```python
from build123d import *

# Parameters (mm, degrees)
BOSS_EXTRUDE1_DEPTH = 2
SKETCH1_3_W         = 42
SKETCH1_3_H         = 2
SKETCH1_3_W_2       = 9
BOSS_EXTRUDE2_DEPTH = 23
FILLET1_R           = 2
SKETCH2_R           = 1.5
CUT_EXTRUDE1_DEPTH  = 25
SKETCH3_R           = 2
SKETCH3_R_2         = 4
SKETCH3_R_3         = 1.5
CUT_EXTRUDE2_DEPTH  = 25
SKETCH4_R           = 2
CUT_EXTRUDE3_DEPTH  = 25


with BuildPart() as part:
    # Sketch1 → Boss-Extrude1 (new body)
    with BuildSketch(Plane.XY):
        with BuildLine():
            Line((-21, -18.5), (21, -18.5))
            Line((21, -18.5), (21, -10.5))
            Line((21, -10.5), (27, -10.5))
            ThreePointArc((27, -10.5), (28.414213562, -9.914213562), (29, -8.5))
            Line((29, -8.5), (29, 14.5))
            Line((29, 14.5), (20, 14.5))
            Line((20, 14.5), (20, 8.5))
            Line((20, 8.5), (18, 8.5))
            Line((18, 8.5), (18, 16.5))
            ThreePointArc((18, 16.5), (17.414213562, 17.914213562), (16, 18.5))
            Line((16, 18.5), (-16, 18.5))
            ThreePointArc((-16, 18.5), (-17.414213562, 17.914213562), (-18, 16.5))
            Line((-18, 16.5), (-18, 8.5))
            Line((-18, 8.5), (-20, 8.5))
            Line((-20, 8.5), (-20, 14.5))
            Line((-20, 14.5), (-29, 14.5))
            Line((-29, 14.5), (-29, -8.5))
            ThreePointArc((-29, -8.5), (-28.414213562, -9.914213562), (-27, -10.5))
            Line((-27, -10.5), (-21, -10.5))
            Line((-21, -10.5), (-21, -18.5))
        make_face()
    extrude(amount=-BOSS_EXTRUDE1_DEPTH)

    # Sketch1<3> → Boss-Extrude2 (add)
    with BuildSketch(Plane.XY):
        with Locations((0, -17.5)):
            Rectangle(SKETCH1_3_W, SKETCH1_3_H)
        with Locations((-24.5, 13.5)):
            Rectangle(SKETCH1_3_W_2, SKETCH1_3_H)
        with Locations((24.5, 13.5)):
            Rectangle(SKETCH1_3_W_2, SKETCH1_3_H)
    extrude(amount=BOSS_EXTRUDE2_DEPTH)

    # Fillet1
    fillet1_edges = [part.edges().sort_by_distance(p)[0] for p in [
        (0, -18.5, -2),
        (24.5, 14.5, -2),
        (21, -17.5, 23),
        (-21, -17.5, 23),
        (-29, 13.5, 23),
        (-20, 13.5, 23),
        (20, 13.5, 23),
        (29, 13.5, 23),
        (-24.5, 14.5, -2),
    ]]
    fillet(fillet1_edges, radius=FILLET1_R)

    # Sketch2 → Cut-Extrude1 (cut)
    with BuildSketch(Plane(origin=(0, -16.5, 0), x_dir=(1, 0, 0), z_dir=(0, 1, 0))):
        with Locations((17.5, -11)):
            Circle(SKETCH2_R)
        with Locations((10.5, -11)):
            Circle(SKETCH2_R)
        with Locations((10.5, -18)):
            Circle(SKETCH2_R)
        with Locations((3.5, -11)):
            Circle(SKETCH2_R)
        with Locations((10.5, -4)):
            Circle(SKETCH2_R)
        with Locations((-17.5, -11)):
            Circle(SKETCH2_R)
        with Locations((-10.5, -18)):
            Circle(SKETCH2_R)
        with Locations((-10.5, -11)):
            Circle(SKETCH2_R)
        with Locations((-3.5, -11)):
            Circle(SKETCH2_R)
        with Locations((-10.5, -4)):
            Circle(SKETCH2_R)
    extrude(amount=-CUT_EXTRUDE1_DEPTH, mode=Mode.SUBTRACT)

    # Sketch3 → Cut-Extrude2 (cut)
    with BuildSketch(Plane.XY):
        with Locations((-24, -4.5)):
            Circle(SKETCH3_R)
        with Locations((-24, 5.5)):
            Circle(SKETCH3_R)
        with Locations((-10, 6.5)):
            Circle(SKETCH3_R_2)
        with Locations((-3, 6.5)):
            Circle(SKETCH3_R_3)
        with Locations((-10, -0.5)):
            Circle(SKETCH3_R_3)
        with Locations((-17, 6.5)):
            Circle(SKETCH3_R_3)
        with Locations((-10, 13.5)):
            Circle(SKETCH3_R_3)
        with Locations((10, -0.5)):
            Circle(SKETCH3_R_3)
        with Locations((3, 6.5)):
            Circle(SKETCH3_R_3)
        with Locations((10, 13.5)):
            Circle(SKETCH3_R_3)
        with Locations((10, 6.5)):
            Circle(SKETCH3_R_2)
        with Locations((17, 6.5)):
            Circle(SKETCH3_R_3)
        with Locations((24, -4.5)):
            Circle(SKETCH3_R)
        with Locations((24, 5.5)):
            Circle(SKETCH3_R)
        with Locations((0, -4.5)):
            Circle(SKETCH3_R_2)
        with Locations((0, -11.5)):
            Circle(SKETCH3_R_3)
        with Locations((-7, -4.5)):
            Circle(SKETCH3_R_3)
        with Locations((0, 2.5)):
            Circle(SKETCH3_R_3)
        with Locations((7, -4.5)):
            Circle(SKETCH3_R_3)
    extrude(amount=-CUT_EXTRUDE2_DEPTH, mode=Mode.SUBTRACT)

    # Sketch4 → Cut-Extrude3 (cut)
    with BuildSketch(Plane(origin=(0, 14.5, 0), x_dir=(1, 0, 0), z_dir=(0, 1, 0))):
        with Locations((-24, -7)):
            Circle(SKETCH4_R)
        with Locations((-24, -17)):
            Circle(SKETCH4_R)
        with Locations((24, -17)):
            Circle(SKETCH4_R)
        with Locations((24, -7)):
            Circle(SKETCH4_R)
    extrude(amount=-CUT_EXTRUDE3_DEPTH, mode=Mode.SUBTRACT)


solid = part.part
```
Verification items for the finished model (mm, model axes). A direction names the side the tool comes from. Give positions to 0.01 mm unless a question says otherwise; leave off trailing zeros. Order: outer loops, then holes, each group sorted by start corner. A loop starts at its lowest first (then second) coordinate and runs counter-clockwise, first axis right, second up. Notation, with made-up numbers: (19, -8.75) -> (32, -8.75) arc R19 ccw to (32, 10.25) -> close; hole circle Ø6 at (30, 9). An arc over 180 degrees is marked (long way). One line per item, written item: value.
(1) Gauge pin test, flat ends, axial feed: pin 1 (5 mm diameter, centred on x = -24, y = 5.5, fed in from +Z); pin 2 (3.5 mm diameter, centred on x = -10.5, z = 11, fed in from +Y); pin 3 (1 mm diameter, centred on x = 25, z = -0.5, fed in from -Y); pin 4 (2.5 mm diameter, centred on x = 10.5, z = 4, fed in from -Y). Record the tip position at first contact, or that the pin passes through.
Final values:
pin 1: z = 0
pin 2: y = -16.5
pin 3: y = -10.5
pin 4: through
(2) Tool access check on faces 1 (the face through (24.44, 13.93, -1.4)), 2 (the face through (20.57, 13.51, 22.4)), 3 (the face through (19, 8.5, -1)). Record the directions out of +Z, -Z, +X, -X, +Y, -Y that give a thin tool (end or side, any length) a straight path to the whole face; none if there is none.
Final values:
face 1: -Z, +X, +Y
face 2: +Z, +Y
face 3: +Z, -Z, +Y
(3) Sectioned sample at B-B on x = -24. Record the cut outline in (y, z), then the cut area to 3 significant figures.
Final values:
outline: (-10.5, -2) -> (-6.5, -2) -> (-6.5, 0) -> (-10.5, 0) -> close; (-2.5, -2) -> (3.5, -2) -> (3.5, 0) -> (-2.5, 0) -> close; (7.5, -2) -> (12.5, -2) arc R2 ccw to (14.5, 0) -> (14.5, 5) -> (12.5, 5) -> (12.5, 0) -> (7.5, 0) -> close; (12.5, 9) -> (14.5, 9) -> (14.5, 15) -> (12.5, 15) -> close; (12.5, 19) -> (14.5, 19) -> (14.5, 23) -> (12.5, 23) -> close
area: 63.1 mm^2
(4) Sectioned sample at A-A on z = 7. Record the cut outline in (x, y).
Final values:
outline: (-29, 12.5) -> (-26, 12.5) -> (-26, 14.5) -> (-29, 14.5) -> close; (-22, 12.5) -> (-20, 12.5) -> (-20, 14.5) -> (-22, 14.5) -> close; (-21, -18.5) -> (21, -18.5) -> (21, -16.5) -> (-21, -16.5) -> close; (20, 12.5) -> (22, 12.5) -> (22, 14.5) -> (20, 14.5) -> close; (26, 12.5) -> (29, 12.5) -> (29, 14.5) -> (26, 14.5) -> close
(5) Sectioned sample at C-C on x = 10. Count the separate pieces of the cut face and the enclosed holes in it, then the cut area to 3 significant figures.
Final values:
separate pieces: 7
enclosed holes: 0
area: 74.2 mm^2
(6) Draft check along X on faces 4 (the face through (5.5, -4.43, -0.99)), 5 (the face through (28.4, -9.93, -0.99)), 6 (the face through (0, -17, 23)). Enter one of: pulls with the +X half, pulls with the -X half, needs draft (parallel to the pull), parting line crosses it, or undercut.
Final values:
face 4: undercut
face 5: pulls with the +X half
face 6: needs draft
(7) Scan lines: line 1 along X through (y, z) = (13, 4); line 2 along Y through (x, z) = (-3, -1.6); line 3 along Z through (x, y) = (14, 9.5). Record each from-to range of solid material in increasing order. Write a range as [from, to].
Final values:
line 1: [-29, -20], [20, 29]
line 2: [-17.7, -7.15], [-1.85, 5], [8, 18.5]
line 3: [-2, 0]
